The model under review builds one solid part; all positions refer to its coordinate system, in mm. A direction names the side the tool comes from. Round coordinates to 2 decimals unless told otherwise and drop trailing zeros. Order: outer loops, then holes, each group sorted by start corner. A loop starts at its lowest first (then second) coordinate and runs counter-clockwise, first axis right, second up. Notation, with made-up numbers: M 27,78.25 L 76,78.25 A27 cw 76,107.25 Z; hole C 23,53.5 d2. An arc over 180 degrees is marked long. Answer as a JSON object with one key per item and string values. Group by question number.
1) Consider section A-A, the plane y = -57. Write out the cut boundary in (x, z).
2) Consider section B-B, the plane x = 204. Write out the cut boundary in (y, z), then the cut area to 3 significant figures.
3) The part is to be moulded in two halves that separate along Y. For faces 3 (the flat face through (222, -51, 0)), 4 (the flat face through (215.433, -46.96, 4.93)), 5 (the cylindrical face through (263.9, -7.43, 0.49)), 6 (the flat face through (221, -52, 1)), say which applies: +Y half, -Y half, draft (parallel to the pull), parting line (faces both ways), or undercut.
4) For faces 1 (the flat face through (225.33, -56.86, 4.94)), 2 (the cylindrical face through (178.833, -96.258, 0.493)), list the 3-axis set-ups (+Z, -Z, +X, -X, +Y, -Y) from which the entire face can be reached by the end or side of a thin tool; tool diameter is ignored.
5) To check wall thickness, follow line 1 (Z direction, x = 264, y = -6); line 2 (Y direction, x = 223, z = 8); line 3 (X direction, y = -50.5, z = 3.5). State the ranges of each line that lie inside material, in increasing order.
6) Insertion check: pin 1 Ø1 at (y, z) = (-43, 2) entering from +X; pin 2 Ø1 at (x, z) = (211, 6.5) entering from -Y; pin 3 Ø3 at (x, y) = (177.36, -95.64) entering from -Z; pin 4 Ø1.5 at (x, z) = (199, 4) entering from +Y. Each pin has a flat end and moves straight along its axis. Give the tip position at first contact, or say it passes through.
```python
from build123d import *

# Parameters (mm, degrees)
SKETCH_1_R          = 1.6
EXTRUDE_1_DEPTH     = 10
SKETCH_2_R          = 1.6
CUT_EXTRUDE_1_DEPTH = 20
SKETCH_3_W          = 8
SKETCH_3_H          = 13
CUT_EXTRUDE_2_DEPTH = 1000


with BuildPart() as part:
    # ｽｹｯﾁ1 → ﾎﾞｽ - 押し出し1 (new body)
    with BuildSketch(Plane.XY):
        Polygon((177.355249325, -106.251352393), (166.748647607, -95.644750675), (265.5, 3.106601718), (276.106601718, -7.5), align=None)
        with Locations((265.5, -7.5)):
            Circle(SKETCH_1_R, mode=Mode.SUBTRACT)
        with Locations((177.355249325, -95.644750675)):
            Circle(SKETCH_1_R, mode=Mode.SUBTRACT)
    extrude(amount=EXTRUDE_1_DEPTH)

    # ｽｹｯﾁ2 → ｶｯﾄ - 押し出し1 (cut)
    with BuildSketch(Plane(origin=(131.196699141, -131.196699141, 0), x_dir=(0.7071067811865585, 0.7071067811865366, 0), z_dir=(-0.7071067811865366, 0.7071067811865585, 0))):
        with Locations(Location((70.278047689, -5, 0), (0, 0, 180))):
            Circle(SKETCH_2_R)
    extrude(amount=-CUT_EXTRUDE_1_DEPTH, mode=Mode.SUBTRACT)

    # ｽｹｯﾁ3 → ｶｯﾄ - 押し出し2 (cut)
    with BuildSketch(Plane(origin=(35.551948466, 35.551948466, 0), x_dir=(0, 0, 1), z_dir=(-0.7071067811865581, -0.7071067811865369, 0))):
        with Locations((5, -193.040151264)):
            Rectangle(SKETCH_3_W, SKETCH_3_H)
    extrude(amount=-CUT_EXTRUDE_2_DEPTH, mode=Mode.SUBTRACT)


solid = part.part
```
Results list:
{
 "1": {"outline": "M 205.39,0 L 226.61,0 L 226.61,10 L 205.39,10 Z; hole M 206.81,1 L 225.19,1 L 225.19,9 L 206.81,9 Z"},
 "2": {"outline": "M -79.61,0 L -58.39,0 L -58.39,10 L -79.61,10 Z; hole M -78.19,1 L -59.81,1 L -59.81,9 L -78.19,9 Z", "area": "65.1 mm^2"},
 "3": {"face 3": "draft", "face 4": "+Y half", "face 5": "undercut", "face 6": "undercut"},
 "4": {"face 1": "none", "face 2": "+Z, -Z"},
 "5": {"line 1": "0 to 1, 9 to 10", "line 2": "-60.61 to -59.19, -40.81 to -39.39", "line 3": "211.89 to 213.31, 231.69 to 233.11"},
 "6": {"pin 1": "x = 241.11", "pin 2": "y = -73.11", "pin 3": "through", "pin 4": "y = -62.64"}
}
